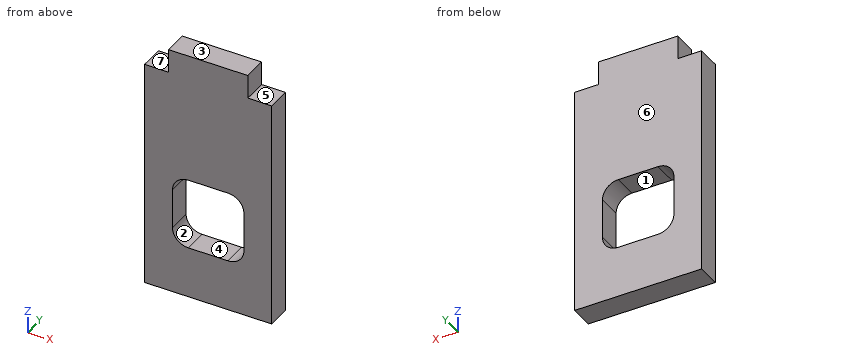
from build123d import *

# Parameters (mm, degrees)
SKETCH1_W               = 16
SKETCH1_H               = 29
BOSS_EXTRUDE1_DEPTH     = 1.5
SKETCH2_W               = 10
SKETCH2_H               = 3
BOSS_EXTRUDE2_DEPTH     = 1.5
SKETCH3_W               = 9
SKETCH3_H               = 9
CUT_EXTRUDE1_DEPTH      = 2.5
CUT_EXTRUDE1_DEPTH_BACK = 2.5
FILLET1_R               = 2


with BuildPart() as part:
    # Sketch1 → Boss-Extrude1 (new body, symmetric)
    with BuildSketch(Plane(origin=(0, 0, 0), x_dir=(1, 0, 0), z_dir=(0, 1, 0))):
        Rectangle(SKETCH1_W, SKETCH1_H)
    extrude(amount=BOSS_EXTRUDE1_DEPTH, both=True)

    # Sketch2 → Boss-Extrude2 (add, symmetric)
    with BuildSketch(Plane(origin=(0, 0, 0), x_dir=(1, 0, 0), z_dir=(0, 1, 0))):
        with Locations((0, -16)):
            Rectangle(SKETCH2_W, SKETCH2_H)
    extrude(amount=BOSS_EXTRUDE2_DEPTH, both=True)

    # Sketch3 → Cut-Extrude1 (cut, two sides)
    with BuildSketch(Plane(origin=(0, 0, 0), x_dir=(1, 0, 0), z_dir=(0, 1, 0))) as cut_extrude1_sk:
        with Locations((0, 3.5)):
            Rectangle(SKETCH3_W, SKETCH3_H)
    extrude(amount=CUT_EXTRUDE1_DEPTH, mode=Mode.SUBTRACT)
    extrude(cut_extrude1_sk.sketch, amount=-CUT_EXTRUDE1_DEPTH_BACK, mode=Mode.SUBTRACT)

    # Fillet1
    fillet1_edges = [part.edges().sort_by_distance(p)[0] for p in [
        (-4.5, 0, 1),
        (-4.5, 0, -8),
        (4.5, 0, -8),
        (4.5, 0, 1),
    ]]
    fillet(fillet1_edges, radius=FILLET1_R)


solid = part.part
Could you check a few things on this model? Use its own coordinates, in mm. Face numbers are marked on the shaded views. A direction names the side the tool comes from. Give positions to 0.01 mm unless a question says otherwise; leave off trailing zeros. Order: outer loops, then holes, each group sorted by start corner. A loop starts at its lowest first (then second) coordinate and runs counter-clockwise, first axis right, second up.
1. Suppose I cut it at A-A (z = -3). Write out the boundary of the cut face in (x, y), plus the area to 3 significant figures.
Answers below:
outline: (-8, -1.5) - (-4.5, -1.5) - (-4.5, 1.5) - (-8, 1.5) - close; (4.5, -1.5) - (8, -1.5) - (8, 1.5) - (4.5, 1.5) - close
area: 21.0 mm2
2. For pin 1 (1.5 mm diameter, centred on x = -6, y = -0.5, fed in from +Z), with a flat end and sliding along its axis, tell me the tip position at first contact or that it passes through.
Answers below:
pin 1: stops at z = 14.5
3. Thinking about a two-plate mould opening in X: for the marked faces 1, 2 and 3, which applies, +X half, -X half, draft (parallel to the pull), parting line (faces both ways), or undercut?
Answers below:
face 1: undercut
face 2: undercut
face 3: draft
4. Suppose I cut it at C-C (y = 0.2). Write out the boundary of the cut face in (x, z).
Answers below:
outline: (-8, -14.5) - (8, -14.5) - (8, 14.5) - (5, 14.5) - (5, 17.5) - (-5, 17.5) - (-5, 14.5) - (-8, 14.5) - close; hole (-4.5, -6) arc R2 ccw to (-2.5, -8) - (2.5, -8) arc R2 ccw to (4.5, -6) - (4.5, -1) arc R2 ccw to (2.5, 1) - (-2.5, 1) arc R2 ccw to (-4.5, -1) - close
5. I need wall thicknesses on L1, parallel to Z at x = 0.5, y = 0.2; L2, parallel to X at y = -1.3, z = 16; L3, parallel to Z at x = -6.75, y = -1.05. Which ranges of each line are inside material? Lowest first, please.
Answers below:
L1: z = -14.5 to -8, 1 to 17.5
L2: x = -5 to 5
L3: z = -14.5 to 14.5
6. Suppose I cut it at D-D (x = 6). Write out the boundary of the cut face in (y, z), plus the area to 3 significant figures.
Answers below:
outline: (-1.5, -14.5) - (1.5, -14.5) - (1.5, 14.5) - (-1.5, 14.5) - close
area: 87.0 mm2
7. Which directions (+Z, -Z, +X, -X, +Y, -Y) give clear straight access to the entire face, cutting with the end or side of a thin tool? Please do the marked faces 4, 5, 6 and 7.
Answers below:
face 4: +Y, -Y
face 5: +Z, +X, +Y, -Y
face 6: +Z, -Z, +X, -X, +Y
face 7: +Z, -X, +Y, -Y
8. Suppose I cut it at B-B (x = -1.75). Write out the boundary of the cut face in (y, z), plus the area to 3 significant figures.
Answers below:
outline: (-1.5, -14.5) - (1.5, -14.5) - (1.5, -8) - (-1.5, -8) - close; (-1.5, 1) - (1.5, 1) - (1.5, 17.5) - (-1.5, 17.5) - close
area: 69.0 mm2
